Part print with two shaded views. Sizes in mm from the minimum x, y, z corner. Round coordinates to 2 decimals unless told otherwise and drop trailing zeros. Order: outer loops, then holes, each group sorted by start corner. A loop starts at its lowest first (then second) coordinate and runs counter-clockwise, first axis right, second up. Notation, with made-up numbers: (71.5, -24.75) - (122.5, -24.75) arc R33 ccw to (122.5, 3.25) - close; hole circle Ø11 at (51.5, -16.5). An arc over 180 degrees is marked (long way). Write item = value, one per line.
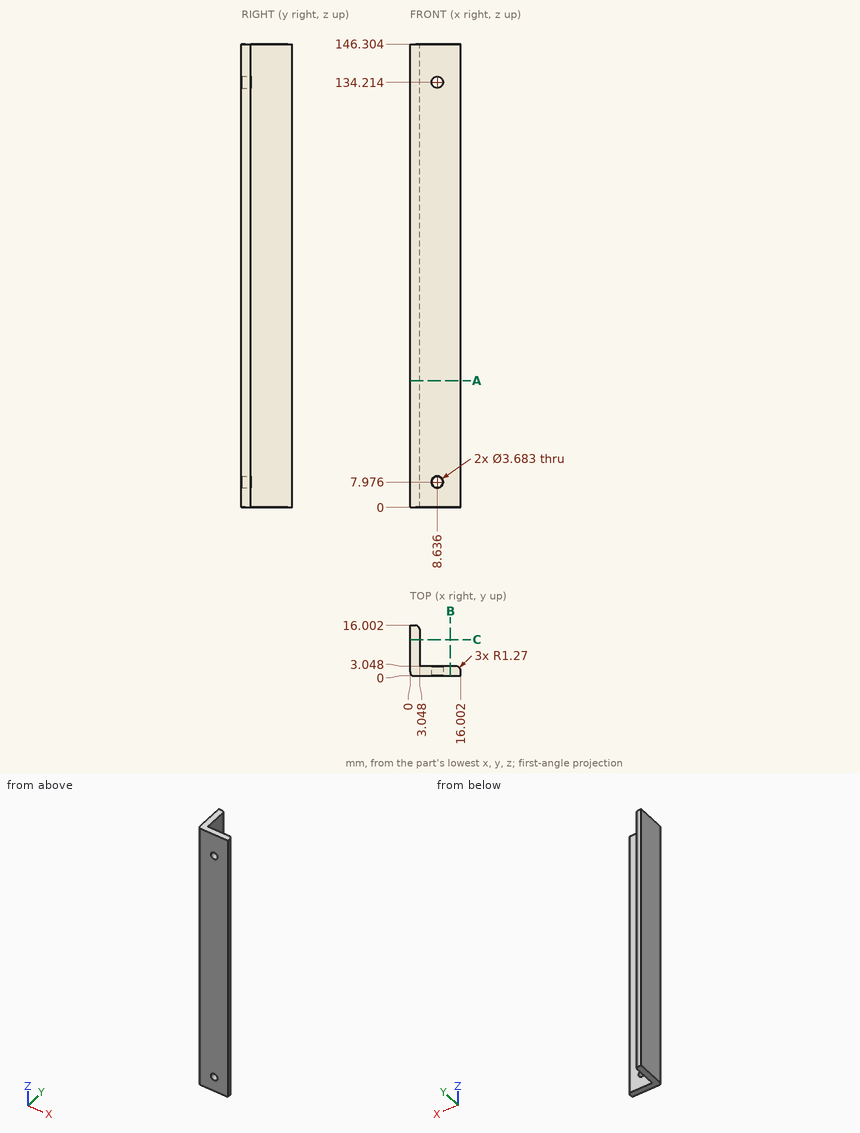
1) Cut at A-A (z = 40). Write the cut outline in (x, y).
Conclusion:
outline = (0, 1.27) arc R1.27 ccw to (1.27, 0) - (16, 0) - (16, 1.78) arc R1.27 ccw to (14.73, 3.05) - (3.05, 3.05) - (3.05, 14.73) arc R1.27 ccw to (1.78, 16) - (0, 16) - close
2) Flat gauge pins, fed straight in: pin 1 Ø3 at (x, y) = (12, 6.5) entering from +Z; pin 2 Ø6 at (x, z) = (8.5, 127.5) entering from +Y; pin 3 Ø4 at (y, z) = (7, 26) entering from +X. Where does each tip first touch, or does it go through?
Conclusion:
pin_1 = through
pin_2 = 3.05
pin_3 = 3.05
3) Cut at B-B (x = 12.75). Write the cut outline in (y, z).
Conclusion:
outline = (0, 0) - (3.05, 0) - (3.05, 146.3) - (0, 146.3) - close
4) Wall check: line 1 along X through (y, z) = (10, 85.5); line 2 along Y through (x, z) = (1, 127.5). Give the ranges that are in metal, low to high.
Conclusion:
line_1 = 0 to 3.05
line_2 = 0.03 to 16
